Here's how the part is built. I have some questions about the finished solid (model axes, mm). A direction names the side the tool comes from. Give positions to 0.01 mm unless a question says otherwise; leave off trailing zeros. Write each loop counter-clockwise with the first axis right and the second up, starting at its lowest first coordinate (ties: lowest second). Pieces come first, ordered by that corner, then holes. Notation, with made-up numbers: (44.25, 38) -> (89.25, 38) arc R23 ccw to (89.25, 46) -> close; hole circle Ø5 at (-35.5, 84). An arc over 180 degrees is marked (long way). Put each result on its own line as item: value. Start each with the question number.
from build123d import *

# Parameters (mm, degrees)
BOSS_EXTRUDE1_DEPTH = 1168.4
CUT_EXTRUDE1_REACH  = 27.4
SKETCH2_R           = 3.175
CUT_EXTRUDE2_REACH  = 5.175
SKETCH3_R           = 1.5875
SKETCH4_R           = 2.667
CUT_EXTRUDE3_DEPTH  = 51.8


with BuildPart() as part:
    # Sketch1 → Boss-Extrude1 (new body)
    with BuildSketch(Plane(origin=(0, 0, 0), x_dir=(1, 0, 0), z_dir=(0, 1, 0))):
        Polygon((3.175, 3.175), (3.175, 25.4), (0, 25.4), (0, 0), (50.8, 0), (50.8, 25.4), (47.625, 25.4), (47.625, 3.175), align=None)
    extrude(amount=BOSS_EXTRUDE1_DEPTH)

    # Sketch2 → Cut-Extrude1 (cut, up to next)
    with BuildSketch(Plane.XY, mode=Mode.PRIVATE) as cut_extrude1_sk1:
        with Locations((25.4, 50.8)):
            Circle(SKETCH2_R)
    cut_extrude1_tool1 = extrude(cut_extrude1_sk1.sketch, amount=-CUT_EXTRUDE1_REACH, mode=Mode.PRIVATE) & part.part
    add(cut_extrude1_tool1.solids().sort_by_distance((25.4, 50.8, 0))[0], mode=Mode.SUBTRACT)
    # Sketch2 → Cut-Extrude1 (cut, up to next)
    with BuildSketch(Plane.XY, mode=Mode.PRIVATE) as cut_extrude1_sk2:
        with Locations((25.4, 152.4)):
            Circle(SKETCH2_R)
    cut_extrude1_tool2 = extrude(cut_extrude1_sk2.sketch, amount=-CUT_EXTRUDE1_REACH, mode=Mode.PRIVATE) & part.part
    add(cut_extrude1_tool2.solids().sort_by_distance((25.4, 152.4, 0))[0], mode=Mode.SUBTRACT)
    # Sketch2 → Cut-Extrude1 (cut, up to next)
    with BuildSketch(Plane.XY, mode=Mode.PRIVATE) as cut_extrude1_sk3:
        with Locations((25.4, 254)):
            Circle(SKETCH2_R)
    cut_extrude1_tool3 = extrude(cut_extrude1_sk3.sketch, amount=-CUT_EXTRUDE1_REACH, mode=Mode.PRIVATE) & part.part
    add(cut_extrude1_tool3.solids().sort_by_distance((25.4, 254, 0))[0], mode=Mode.SUBTRACT)
    # Sketch2 → Cut-Extrude1 (cut, up to next)
    with BuildSketch(Plane.XY, mode=Mode.PRIVATE) as cut_extrude1_sk4:
        with Locations((25.4, 355.6)):
            Circle(SKETCH2_R)
    cut_extrude1_tool4 = extrude(cut_extrude1_sk4.sketch, amount=-CUT_EXTRUDE1_REACH, mode=Mode.PRIVATE) & part.part
    add(cut_extrude1_tool4.solids().sort_by_distance((25.4, 355.6, 0))[0], mode=Mode.SUBTRACT)
    # Sketch2 → Cut-Extrude1 (cut, up to next)
    with BuildSketch(Plane.XY, mode=Mode.PRIVATE) as cut_extrude1_sk5:
        with Locations((25.4, 457.2)):
            Circle(SKETCH2_R)
    cut_extrude1_tool5 = extrude(cut_extrude1_sk5.sketch, amount=-CUT_EXTRUDE1_REACH, mode=Mode.PRIVATE) & part.part
    add(cut_extrude1_tool5.solids().sort_by_distance((25.4, 457.2, 0))[0], mode=Mode.SUBTRACT)
    # Sketch2 → Cut-Extrude1 (cut, up to next)
    with BuildSketch(Plane.XY, mode=Mode.PRIVATE) as cut_extrude1_sk6:
        with Locations((25.4, 558.8)):
            Circle(SKETCH2_R)
    cut_extrude1_tool6 = extrude(cut_extrude1_sk6.sketch, amount=-CUT_EXTRUDE1_REACH, mode=Mode.PRIVATE) & part.part
    add(cut_extrude1_tool6.solids().sort_by_distance((25.4, 558.8, 0))[0], mode=Mode.SUBTRACT)
    # Sketch2 → Cut-Extrude1 (cut, up to next)
    with BuildSketch(Plane.XY, mode=Mode.PRIVATE) as cut_extrude1_sk7:
        with Locations((25.4, 660.4)):
            Circle(SKETCH2_R)
    cut_extrude1_tool7 = extrude(cut_extrude1_sk7.sketch, amount=-CUT_EXTRUDE1_REACH, mode=Mode.PRIVATE) & part.part
    add(cut_extrude1_tool7.solids().sort_by_distance((25.4, 660.4, 0))[0], mode=Mode.SUBTRACT)
    # Sketch2 → Cut-Extrude1 (cut, up to next)
    with BuildSketch(Plane.XY, mode=Mode.PRIVATE) as cut_extrude1_sk8:
        with Locations((25.4, 762)):
            Circle(SKETCH2_R)
    cut_extrude1_tool8 = extrude(cut_extrude1_sk8.sketch, amount=-CUT_EXTRUDE1_REACH, mode=Mode.PRIVATE) & part.part
    add(cut_extrude1_tool8.solids().sort_by_distance((25.4, 762, 0))[0], mode=Mode.SUBTRACT)
    # Sketch2 → Cut-Extrude1 (cut, up to next)
    with BuildSketch(Plane.XY, mode=Mode.PRIVATE) as cut_extrude1_sk9:
        with Locations((25.4, 863.6)):
            Circle(SKETCH2_R)
    cut_extrude1_tool9 = extrude(cut_extrude1_sk9.sketch, amount=-CUT_EXTRUDE1_REACH, mode=Mode.PRIVATE) & part.part
    add(cut_extrude1_tool9.solids().sort_by_distance((25.4, 863.6, 0))[0], mode=Mode.SUBTRACT)
    # Sketch2 → Cut-Extrude1 (cut, up to next)
    with BuildSketch(Plane.XY, mode=Mode.PRIVATE) as cut_extrude1_sk10:
        with Locations((25.4, 965.2)):
            Circle(SKETCH2_R)
    cut_extrude1_tool10 = extrude(cut_extrude1_sk10.sketch, amount=-CUT_EXTRUDE1_REACH, mode=Mode.PRIVATE) & part.part
    add(cut_extrude1_tool10.solids().sort_by_distance((25.4, 965.2, 0))[0], mode=Mode.SUBTRACT)
    # Sketch2 → Cut-Extrude1 (cut, up to next)
    with BuildSketch(Plane.XY, mode=Mode.PRIVATE) as cut_extrude1_sk11:
        with Locations((25.4, 1066.8)):
            Circle(SKETCH2_R)
    cut_extrude1_tool11 = extrude(cut_extrude1_sk11.sketch, amount=-CUT_EXTRUDE1_REACH, mode=Mode.PRIVATE) & part.part
    add(cut_extrude1_tool11.solids().sort_by_distance((25.4, 1066.8, 0))[0], mode=Mode.SUBTRACT)

    # Sketch3 → Cut-Extrude2 (cut, up to next)
    with BuildSketch(Plane(origin=(0, 0, -3.175), x_dir=(-1, 0, 0), z_dir=(0, 0, -1)), mode=Mode.PRIVATE) as cut_extrude2_sk1:
        with Locations((-25.4, 25.4)):
            Circle(SKETCH3_R)
    cut_extrude2_tool1 = extrude(cut_extrude2_sk1.sketch, amount=-CUT_EXTRUDE2_REACH, mode=Mode.PRIVATE) & part.part
    add(cut_extrude2_tool1.solids().sort_by_distance((25.4, 25.4, -3.175))[0], mode=Mode.SUBTRACT)
    # Sketch3 → Cut-Extrude2 (cut, up to next)
    with BuildSketch(Plane(origin=(0, 0, -3.175), x_dir=(-1, 0, 0), z_dir=(0, 0, -1)), mode=Mode.PRIVATE) as cut_extrude2_sk2:
        with Locations((-25.4, 66.020295879)):
            Circle(SKETCH3_R)
    cut_extrude2_tool2 = extrude(cut_extrude2_sk2.sketch, amount=-CUT_EXTRUDE2_REACH, mode=Mode.PRIVATE) & part.part
    add(cut_extrude2_tool2.solids().sort_by_distance((25.4, 66.020296, -3.175))[0], mode=Mode.SUBTRACT)
    # Sketch3 → Cut-Extrude2 (cut, up to next)
    with BuildSketch(Plane(origin=(0, 0, -3.175), x_dir=(-1, 0, 0), z_dir=(0, 0, -1)), mode=Mode.PRIVATE) as cut_extrude2_sk3:
        with Locations((-25.4, 106.640591758)):
            Circle(SKETCH3_R)
    cut_extrude2_tool3 = extrude(cut_extrude2_sk3.sketch, amount=-CUT_EXTRUDE2_REACH, mode=Mode.PRIVATE) & part.part
    add(cut_extrude2_tool3.solids().sort_by_distance((25.4, 106.640592, -3.175))[0], mode=Mode.SUBTRACT)

    # Sketch4 → Cut-Extrude3 (cut, through all)
    with BuildSketch(Plane.ZY):
        with Locations((-15.875, 6.35)):
            Circle(SKETCH4_R)
    extrude(amount=-CUT_EXTRUDE3_DEPTH, mode=Mode.SUBTRACT)


solid = part.part
1) I want a section at A-A, the plane y = 296.5. Write out the boundary of the cut face in (x, z) (3 decimals).
2) Which directions (+Z, -Z, +X, -X, +Y, -Y) give clear straight access to the entire face, cutting with the end or side of a thin tool? Please do faces 4 (the flat face through (25, 576, 0)), 5 (the flat face through (26, 576, -3.175)).
3) I'm going to push a flat-ended pin straight in: pin 1 Ø22 at (x, y) = (25, 443.5) entering from -Z (3 decimals). Where does the tip first touch, or does it pass through?
4) I want a section at B-B, the plane x = 13.5. Write out the boundary of the cut face in (y, z) (3 decimals).
5) Thinking about a two-plate mould opening in X: for faces 1 (the flat face through (50.8, 576, -13)), 2 (the flat face through (0, 576, -13)), 3 (the flat face through (47.625, 576, -14)), which applies, released by +X, released by -X, zero draft, split by the parting line, or undercut?
6) I need wall thicknesses on probe 1 along X at (y, z) = (602.5, -5.25) (3 decimals); probe 2 along X at (y, z) = (863.6, -2) (3 decimals); probe 3 along Z at (x, y) = (14, 866.5) (3 decimals). Which ranges of each line are inside material? Lowest first, please.
Established:
1. outline: (0, -25.4) -> (3.175, -25.4) -> (3.175, -3.175) -> (47.625, -3.175) -> (47.625, -25.4) -> (50.8, -25.4) -> (50.8, 0) -> (0, 0) -> close
2. face 4: +Z, +X, -X, +Y, -Y
2. face 5: -Z, +Y, -Y
3. pin 1: stops at z = -3.175
4. outline: (0, -3.175) -> (1168.4, -3.175) -> (1168.4, 0) -> (0, 0) -> close
5. face 1: released by +X
5. face 2: released by -X
5. face 3: undercut
6. probe 1: x = 0 to 3.175, 47.625 to 50.8
6. probe 2: x = 0 to 22.225, 28.575 to 50.8
6. probe 3: z = -3.175 to 0
